from build123d import *

# Parameters (mm, degrees)
SKETCH2_R           = 3.175
SKETCH2_R_2         = 4.7625
SKETCH2_W           = 16.516490401
SKETCH2_H           = 89.916
SKETCH2_W_2         = 10.16
SKETCH2_H_2         = 63.685061478
SKETCH2_H_3         = 63.685061479
BOSS_EXTRUDE1_DEPTH = 10


with BuildPart() as part:
    # Sketch2 → Boss-Extrude1 (new body)
    with BuildSketch(Plane.XY):
        with BuildLine():
            Line((-408.921789204, 152.75736057), (-459.721789204, 152.75736057))
            Line((-459.721789204, 152.75736057), (-459.721789204, -230.78263943))
            ThreePointArc((-459.721789204, -230.78263943), (-437.403325931, -284.664176156), (-383.521789204, -306.98263943))
            Line((-383.521789204, -306.98263943), (-303.521789204, -306.98263943))
            Line((-303.521789204, -306.98263943), (-303.521789204, -317.14263943))
            Line((-303.521789204, -317.14263943), (-252, -317.14263943))
            Line((-252, -317.14263943), (-252, -306.98263943))
            Line((-252, -306.98263943), (-200.66, -306.98263943))
            Line((-200.66, -306.98263943), (-200.66, -243.280152529))
            Line((-200.66, -243.280152529), (-190.5, -243.280152529))
            Line((-190.5, -243.280152529), (-190.5, -306.98263943))
            Line((-190.5, -306.98263943), (-168.529, -306.98263943))
            Line((-168.529, -306.98263943), (-168.529, -192.68263943))
            Line((-168.529, -192.68263943), (168.529, -192.68263943))
            Line((168.529, -192.68263943), (168.529, -306.98263943))
            Line((168.529, -306.98263943), (190.5, -306.98263943))
            Line((190.5, -306.98263943), (190.5, -243.280152529))
            Line((190.5, -243.280152529), (200.66, -243.280152529))
            Line((200.66, -243.280152529), (200.66, -306.98263943))
            Line((200.66, -306.98263943), (252, -306.98263943))
            Line((252, -306.98263943), (252, -317.14263943))
            Line((252, -317.14263943), (303.521789204, -317.14263943))
            Line((303.521789204, -317.14263943), (303.521789204, -306.98263943))
            Line((303.521789204, -306.98263943), (383.521789204, -306.98263943))
            ThreePointArc((383.521789204, -306.98263943), (437.403325931, -284.664176156), (459.721789204, -230.78263943))
            Line((459.721789204, -230.78263943), (459.721789204, 152.75736057))
            Line((459.721789204, 152.75736057), (408.921789204, 152.75736057))
            Line((408.921789204, 152.75736057), (408.921789204, 142.59736057))
            Line((408.921789204, 142.59736057), (332.721789204, 142.59736057))
            Line((332.721789204, 142.59736057), (332.721789204, 152.75736057))
            Line((332.721789204, 152.75736057), (134.539041792, 152.75736057))
            Line((134.539041792, 152.75736057), (101.6, 317.14263943))
            Line((101.6, 317.14263943), (-101.6, 317.14263943))
            Line((-101.6, 317.14263943), (-134.539041792, 152.75736057))
            Line((-134.539041792, 152.75736057), (-332.721789204, 152.75736057))
            Line((-332.721789204, 152.75736057), (-332.721789204, 142.597360571))
            Line((-332.721789204, 142.597360571), (-408.921789204, 142.597360571))
            Line((-408.921789204, 142.597360571), (-408.921789204, 152.75736057))
        make_face()
        with Locations((368.427, -265.98703943)):
            Circle(SKETCH2_R, mode=Mode.SUBTRACT)
        with Locations((368.427, -240.58703943)):
            Circle(SKETCH2_R, mode=Mode.SUBTRACT)
        with Locations((336.550272189, -94.687385458)):
            Circle(SKETCH2_R, mode=Mode.SUBTRACT)
        with Locations((378.573819589, -5.78737531)):
            Circle(SKETCH2_R, mode=Mode.SUBTRACT)
        with Locations((336.550272189, -5.787385458)):
            Circle(SKETCH2_R, mode=Mode.SUBTRACT)
        with Locations((336.550272189, 83.112614542)):
            Circle(SKETCH2_R, mode=Mode.SUBTRACT)
        with Locations((412.750272189, 83.112614542)):
            Circle(SKETCH2_R, mode=Mode.SUBTRACT)
        with Locations((-412.75027219, 83.112614542)):
            Circle(SKETCH2_R, mode=Mode.SUBTRACT)
        with Locations((-336.55027219, 83.112614542)):
            Circle(SKETCH2_R, mode=Mode.SUBTRACT)
        with Locations((-336.55027219, -5.787385458)):
            Circle(SKETCH2_R, mode=Mode.SUBTRACT)
        with Locations((-378.573819589, -5.78737531)):
            Circle(SKETCH2_R, mode=Mode.SUBTRACT)
        with Locations((-336.55027219, -94.687385458)):
            Circle(SKETCH2_R, mode=Mode.SUBTRACT)
        with Locations((-368.427, -240.58703943)):
            Circle(SKETCH2_R, mode=Mode.SUBTRACT)
        with Locations((-368.427, -265.98703943)):
            Circle(SKETCH2_R, mode=Mode.SUBTRACT)
        with Locations((172.2755, 127.35736057)):
            Circle(SKETCH2_R_2, mode=Mode.SUBTRACT)
        with Locations((172.2755, 25.75736057)):
            Circle(SKETCH2_R_2, mode=Mode.SUBTRACT)
        with Locations((81.7245, 25.75736057)):
            Circle(SKETCH2_R_2, mode=Mode.SUBTRACT)
        with Locations((81.7245, 127.35736057)):
            Circle(SKETCH2_R_2, mode=Mode.SUBTRACT)
        with Locations((-81.7245, 25.75736057)):
            Circle(SKETCH2_R_2, mode=Mode.SUBTRACT)
        with Locations((-81.7245, 127.35736057)):
            Circle(SKETCH2_R_2, mode=Mode.SUBTRACT)
        with Locations((-172.2755, 127.35736057)):
            Circle(SKETCH2_R_2, mode=Mode.SUBTRACT)
        with Locations((-172.2755, 25.75736057)):
            Circle(SKETCH2_R_2, mode=Mode.SUBTRACT)
        with Locations((0, -78.38263943)):
            Circle(SKETCH2_R, mode=Mode.SUBTRACT)
        with Locations((-95.25, -84.73263943)):
            Circle(SKETCH2_R_2, mode=Mode.SUBTRACT)
        with Locations((95.25, -84.73263943)):
            Circle(SKETCH2_R_2, mode=Mode.SUBTRACT)
        with Locations((312.416754739, 7.72336057)):
            Rectangle(SKETCH2_W, SKETCH2_H, mode=Mode.SUBTRACT)
        with Locations((312.416754739, -172.10863943)):
            Rectangle(SKETCH2_W, SKETCH2_H, mode=Mode.SUBTRACT)
        with Locations((-312.416754739, -172.10863943)):
            Rectangle(SKETCH2_W, SKETCH2_H, mode=Mode.SUBTRACT)
        with Locations((-312.416754739, 7.72336057)):
            Rectangle(SKETCH2_W, SKETCH2_H, mode=Mode.SUBTRACT)
        with Locations((195.58, -147.752560311)):
            Rectangle(SKETCH2_W_2, SKETCH2_H_2, mode=Mode.SUBTRACT)
        with Locations((195.58, -20.382437355)):
            Rectangle(SKETCH2_W_2, SKETCH2_H_3, mode=Mode.SUBTRACT)
        with Locations((195.58, 106.97026018)):
            Rectangle(SKETCH2_W_2, SKETCH2_H_3, mode=Mode.SUBTRACT)
        with Locations((-195.58, 106.97026018)):
            Rectangle(SKETCH2_W_2, SKETCH2_H_3, mode=Mode.SUBTRACT)
        with Locations((-195.58, -20.382437355)):
            Rectangle(SKETCH2_W_2, SKETCH2_H_3, mode=Mode.SUBTRACT)
        with Locations((-195.58, -147.752560311)):
            Rectangle(SKETCH2_W_2, SKETCH2_H_2, mode=Mode.SUBTRACT)
    extrude(amount=-BOSS_EXTRUDE1_DEPTH)


solid = part.part
Geometry: final body of the model. Coordinates: model frame, mm. Round coordinates to 2 decimals unless told otherwise and drop trailing zeros. Order: outer loops, then holes, each group sorted by start corner. A loop starts at its lowest first (then second) coordinate and runs counter-clockwise, first axis right, second up. Notation, with made-up numbers: (-36.75, -35) -> (11.25, -35) arc R13 ccw to (11.25, -10) -> close; hole circle Ø11 at (80, 21). An arc over 180 degrees is marked (long way). Put each result on its own line as item: value. Start each with the question number.
Q1. Section D-D on x = -125.5. Return the cut outline in (y, z), and give its area (3 significant figures).
Q2. Line query: probe 1 along Y at (x, z) = (200, -2); probe 2 along X at (y, z) = (-15.5, -4.75) (1 decimal); probe 3 along X at (y, z) = (100, -5.75). Output: solid intervals per line, ascending.
Q3. Pull-direction query (Z, two-part tool) for faces 1 (the flat face through (-6, 4, 0)), 2 (the cylindrical face through (-437.99, -284.07, -4.93)), 3 (the flat face through (-6, 4, -10)); classes: +Z half, -Z half, draft (parallel to the pull), parting line (faces both ways), or undercut.
Q4. Section B-B on x = 236.5. Return the cut outline in (y, z).
Q5. First-contact query: pin 1 (5 mm diameter, centred on x = -269, z = -1, fed in from +Y); pin 2 (3 mm diameter, centred on y = -279, z = -4, fed in from +X); pin 3 (3 mm diameter, centred on y = 189.5, z = -1.5, fed in from -X); pin 4 (5.5 mm diameter, centred on x = -172.28, y = 25.76, fed in from -Z). Flat tips, straight axial feed; report the tip coordinate or a pass-through.
Q6. Section C-C on z = -8. Give the number of separate pieces and of enclosed holes in the cut face, and give its area (3 significant figures).
Q7. Section A-A on y = -202. Return the cut outline in (x, z) (1 decimal), and give its area (3 significant figures).
Ans:
1. outline: (-192.68, -10) -> (197.87, -10) -> (197.87, 0) -> (-192.68, 0) -> close
1. area: 3,910 mm2
2. probe 1: y = -243.28 to -179.6, -115.91 to -52.22, 11.46 to 75.13, 138.81 to 152.76
2. probe 2: x = -459.7 to -320.7, -304.2 to -200.7, -190.5 to 190.5, 200.7 to 304.2, 320.7 to 459.7
2. probe 3: x = -459.72 to -200.66, -190.5 to 190.5, 200.66 to 459.72
3. face 1: +Z half
3. face 2: draft
3. face 3: -Z half
4. outline: (-306.98, -10) -> (152.76, -10) -> (152.76, 0) -> (-306.98, 0) -> close
5. pin 1: stops at y = 152.76
5. pin 2: stops at x = 443.72
5. pin 3: stops at x = -127.48
5. pin 4: passes through
6. separate pieces: 1
6. enclosed holes: 35
6. area: 408,000 mm2
7. outline: (-459.7, -10) -> (-320.7, -10) -> (-320.7, 0) -> (-459.7, 0) -> close; (-304.2, -10) -> (-168.5, -10) -> (-168.5, 0) -> (-304.2, 0) -> close; (168.5, -10) -> (304.2, -10) -> (304.2, 0) -> (168.5, 0) -> close; (320.7, -10) -> (459.7, -10) -> (459.7, 0) -> (320.7, 0) -> close
7. area: 5,490 mm2
